Autodesk Inventor part; units mm, degrees
ref_plane "Начальная плоскость" through (0, 0, 65) normal (0, 0, 1) x (1, 0, 0)
ref_plane "Конечная плоскость" through (0, 0, 145) normal (0, 0, 1) x (1, 0, 0)
ref_plane "РабПлоскость8" through (18, 0, 145) normal (0, 0, 1) x (1, 0, 0)
ref_plane "Начальная плоскость" through (0, 0, 65) normal (0, 0, 1) x (1, 0, 0)
ref_plane "Конечная плоскость" through (0, 0, 145) normal (0, 0, 1) x (1, 0, 0)
sketch "Эскиз" plane through (0, 0, 0) normal (0, 0, 1) x (1, 0, 0)
  line L0 (36, -32.5) -> (0, -32.5)
  line L1 (36, -32.5) -> (36, -28.696)
  line L2 (33.6994, -26.2039) -> (9.9215, -24.3017)
  line L3 (4.4, -18.3208) -> (4.4, 18.3208)
  line L4 (33.6994, 26.2039) -> (9.9215, 24.3017)
  line L5 (36, 28.696) -> (36, 32.5)
  line L6 (0, 32.5) -> (36, 32.5)
  line L7 (0, -32.5) -> (0, 32.5)
  arc A0 (4.4, -18.3208) -> (9.9215, -24.3017) centre (10.4, -18.3208) ccw
  arc A1 (9.9215, 24.3017) -> (4.4, 18.3208) centre (10.4, 18.3208) ccw
  arc A2 (36, -28.696) -> (33.6994, -26.2039) centre (33.5, -28.696) ccw
  arc A3 (33.6994, 26.2039) -> (36, 28.696) centre (33.5, 28.696) ccw
  line L8 (0, 45.5) -> (0, -45.5) construction
  line L9 (-7.2974, 0) -> (43.7847, 0) construction
  point P0 (36, -26.388)
  point P1 (4.4, -23.86)
  point P2 (4.4, 23.86)
  point P3 (36, 26.388)
  dimension "d3" = 36
  dimension "d5" = 4.4
  dimension "d7" = 65
  dimension "d9" = 8.64
  dimension "d11" = 8.64
  dimension "d13" = 6.112
  dimension "d15" = 6.112
  dimension "d22" = 6
  dimension "d23" = 2.5
  dimension "d24" = 32.5
  dimension "d25" = 0
extrude "Тело" add sketch "Эскиз" along normal up to surface (80 mm away) from surface at 65
sketch "Sketch3" plane through (0, 0, 0) normal (0, 0, 1) x (1, 0, 0)
  line L0 (0, 0) -> (10, 0)
ref_plane "Work Plane7" through (0, 0, 0) normal (0, -1, 0) x (1, 0, 0)
sketch "Sketch4" plane through (0, 0, 0) normal (0, -1, 0) x (1, 0, 0)
  line L0 (-2, 65) -> (12, 65)
  line L1 (-2, 145) -> (12, 145)
  dimension "d29" = 80
ref_plane "РабПлоскость8" through (18, 0, 145) normal (0, 0, 1) x (1, 0, 0)
split "Разделение1" plane through (18, 0, 145) removes the side toward (0, 0, 1)
ref_plane "РабПлоскость9" through (18, 0, 145) normal (0, 0, 1) x (1, 0, 0)
split "Разделение2" plane through (18, 0, 145) removes the side toward (0, 0, 1)
ref_plane "РабПлоскость10" through (18, 0, 65) normal (0, 0, -1) x (-1, 0, 0)
split "Разделение3" plane through (18, 0, 65) removes the side toward (0, 0, -1)
equation "\"d3\" = b"
equation "\"d7\" = ParH"
equation "\"d22\" = R"
equation "\"d23\" = R1"
equation "\"d24\" = 0.5 * d7"
equation "\"d16\" = G_L"
equation "\"R1\" = 2.5"
equation "\"R\" = 6"
equation "\"t1\" = 4.4"
equation "\"t2\" = 7.2"
equation "\"ParH\" = 65"
equation "\"b\" = 36"
equation "\"msp_x1\" = 0.04 * b"
equation "\"msp_x2\" = -0.08 * t1 + 0.04 * b"
equation "\"G_L\" = d29"
equation "\"ex\" = 0"
equation "\"G_OFFSET_START\" = -65"
equation "\"G_OFFSET_END\" = -65"
equation "\"d26\" = -G_OFFSET_START"
equation "\"d27\" = G_OFFSET_END + B_L"
properties part number "Швеллер 6.5U-80 ГОСТ 8240-97"
The listing builds one solid part. Answer for the finished solid, in the listing's coordinates (mm). A direction names the side the tool comes from. Coordinates: 2 decimals unless noted, no trailing zeros. Write each loop counter-clockwise with the first axis right and the second up, starting at its lowest first coordinate (ties: lowest second). Pieces come first, ordered by that corner, then holes. Notation, with made-up numbers: M 57.25,89.5 L 84.25,89.5 A18 ccw 84.25,113.5 Z; hole C 43,-6 d11. An arc over 180 degrees is marked long. Put each result on its own line as item: value. Start each with the question number.
1. A cutting plane is placed at A-A on x = 7.5. Write down the section's boundary in (y, z).
2. For a pull along Y with two mould halves and no side action, classify faces 1 (the flat face through (18, -32.5, 104)), 2 (the cylindrical face through (5.949, 22.345, 104.44)), 3 (the cylindrical face through (6, -22.4, 104.4)), 4 (the flat face through (18, 32.5, 104)) as pulls with the +Y half, pulls with the -Y half, needs draft (parallel to the pull), parting line crosses it, or undercut.
3. Flat-ended cylindrical pins translate along their axes: P1, Ø4, axis at y = -9, z = 90, coming from the +X side; P2, Ø4, axis at y = 21.5, z = 96, coming from the -X side. Find the tip coordinate at first contact, or state that the pin passes through.
4. A cutting plane is placed at B-B on z = 75.5. Write down the section's boundary in (x, y).
5. A cutting plane is placed at D-D on x = 30. Write down the section's boundary in (y, z).
6. Consider line 1 (Y direction, x = 33.5, z = 133.5); line 2 (Y direction, x = 10, z = 122); line 3 (X direction, y = 8.5, z = 141). Determine where each line is inside the solid, lowest interval first. Write a range as from..to.
7. A cutting plane is placed at C-C on y = -15. Write down the section's boundary in (x, z), then the cut area to 3 significant figures.
8. Which of the six approach directions +Z, -Z, +X, -X, +Y, -Y give full straight-line access (tool end or side, diameter ignored) to faces 5 (the flat face through (21.977, -25.266, 104.44)), 6 (the flat face through (3, 0, 65))?
Resolved:
1. outline: M -32.5,65 L -23.57,65 L -23.57,145 L -32.5,145 Z; M 23.57,65 L 32.5,65 L 32.5,145 L 23.57,145 Z
2. face 1: pulls with the -Y half
2. face 2: undercut
2. face 3: undercut
2. face 4: pulls with the +Y half
3. P1: stops at x = 4.4
3. P2: stops at x = 0
4. outline: M 0,-32.5 L 36,-32.5 L 36,-28.7 A2.5 ccw 33.7,-26.2 L 9.92,-24.3 A6 cw 4.4,-18.32 L 4.4,18.32 A6 cw 9.92,24.3 L 33.7,26.2 A2.5 ccw 36,28.7 L 36,32.5 L 0,32.5 Z
5. outline: M -32.5,65 L -25.91,65 L -25.91,145 L -32.5,145 Z; M 25.91,65 L 32.5,65 L 32.5,145 L 25.91,145 Z
6. line 1: y = -32.5..-26.19, 26.19..32.5
6. line 2: y = -32.5..-24.31, 24.31..32.5
6. line 3: x = 0..4.4
7. outline: M 0,65 L 4.4,65 L 4.4,145 L 0,145 Z
7. area: 352 mm2
8. face 5: +Z, -Z, +X
8. face 6: -Z, +X, -X, +Y, -Y
